Could you check a few things on this model? Use its own coordinates, in mm. A direction names the side the tool comes from. Round coordinates to 2 decimals unless told otherwise and drop trailing zeros. Write each loop counter-clockwise with the first axis right and the second up, starting at its lowest first coordinate (ties: lowest second). Pieces come first, ordered by that corner, then holes. Notation, with made-up numbers: (13.5, 22.25) -> (32.5, 22.25) arc R17 cw to (32.5, 47.25) -> close; hole circle Ø2 at (50.5, -20). An arc over 180 degrees is marked (long way). One line per question, with ' | ' between items. Start each with the question number.
1. For faces 4 (the flat face through (37, 16, 35)), 5 (the flat face through (-37.25, 18, 18)), 6 (the flat face through (-40, 18.5, 9)), which set-ups out of +Z, -Z, +X, -X, +Y, -Y let a thin tool reach every point of the face, with its end or its side?
2. Imagine slicing it at D-D, the plane y = -19. List the corners of the cut face in (x, z) for me.
3. Imagine slicing it at C-C, the plane z = 34. List the corners of the cut face in (x, y) for me.
4. If I drill on line 1 along Z through (x, y) = (-40, 17); line 2 along X through (y, z) = (17, 18); line 3 along X through (y, z) = (16, 9), over which ranges is the centre line in solid material (lowest first)? Write a range as [from, to].
5. For pin 1 Ø5 at (x, y) = (-2, 15.5) entering from +Z; pin 2 Ø8 at (x, y) = (-39.5, 17.5) entering from +Z; pin 3 Ø5 at (x, y) = (-17, 15.5) entering from -Z; pin 4 Ø1.2 at (x, z) = (28, 9) entering from -Y, each with a flat end and sliding along its axis, tell me the tip position at first contact or that it passes through.
6. Imagine slicing it at A-A, the plane x = 20.5. List the corners of the cut face in (y, z) for me, and give its area (3 significant figures).
7. Imagine slicing it at B-B, the plane z = 25.75. List the corners of the cut face in (x, y) for me.
8. Thinking about a two-plate mould opening in Y: for faces 1 (the flat face through (28, 18.5, 26)), 2 (the flat face through (44, 11, 18)), 3 (the flat face through (-7, 17, 3.25)), which applies, released by +Y, released by -Y, zero draft, split by the parting line, or undercut?
from build123d import *

# Parameters (mm, degrees)
F2_DEPTH     = 35
F4_DEPTH     = 10
F3_R         = 2
F5_DEPTH     = 0.95
F6_DEPTH     = 2.5
F7_DEPTH     = 6
F8_W         = 9
F8_H         = 9.25
F8_R         = 1.5
F8_H_2       = 6.25
F9_DEPTH     = 10
F10_DEPTH    = 10
F11_R        = 2
F12_DEPTH    = 6
F13_T1_DEPTH = 35
F13_T3_DEPTH = 35
F13_T5_DEPTH = 60
F13_T7_DEPTH = 32.9128784748


# Not quite as in the source:
# - a fillet or chamfer that OpenCascade refuses, or shapes differently, is made with other operations: its cross-section is extruded or revolved along the edge and cut away or added


with BuildPart() as f2:
    # F1 (on Top) → F2 (new body)
    with BuildSketch(Plane.XY):
        Polygon((50, -22.5), (50, 22.5), (-50, 22.5), (-50, 12.5), (40, 12.5), (40, -22.5), align=None)
    extrude(amount=F2_DEPTH)

    # F3 (on face) → F4 (cut, through all)
    with BuildSketch(Plane.XZ.offset(-12.5)):
        with BuildLine():
            Line((-37.25, 3.25), (24.75, 3.25))
            Line((24.75, 3.25), (24.75, 16.5))
            ThreePointArc((24.75, 16.5), (23.75, 17.5), (24.75, 18.5))
            Line((24.75, 18.5), (24.75, 31.75))
            Line((24.75, 31.75), (-37.25, 31.75))
            Line((-37.25, 31.75), (-37.25, 18.5))
            ThreePointArc((-37.25, 18.5), (-36.25, 17.5), (-37.25, 16.5))
            Line((-37.25, 16.5), (-37.25, 3.25))
        make_face()
        with BuildLine():
            Line((-37.25, 17.5), (-37.25, 16.5))
            ThreePointArc((-37.25, 16.5), (-36.25, 17.5), (-37.25, 18.5))
            Line((-37.25, 18.5), (-37.25, 17.5))
        make_face()
        with BuildLine():
            ThreePointArc((24.75, 18.5), (23.75, 17.5), (24.75, 16.5))
            Line((24.75, 16.5), (24.75, 17.5))
            Line((24.75, 17.5), (24.75, 18.5))
        make_face()
    extrude(amount=-F4_DEPTH, mode=Mode.SUBTRACT)

    # F3 (on face) → F5 (cut)
    with BuildSketch(Plane.XZ.offset(-12.5)):
        with BuildLine():
            Line((-43.25, 3.25), (-37.25, 3.25))
            Line((-37.25, 3.25), (-37.25, 16.5))
            Line((-37.25, 16.5), (-40.25, 16.5))
            ThreePointArc((-40.25, 16.5), (-41.25, 17.5), (-40.25, 18.5))
            Line((-40.25, 18.5), (-37.25, 18.5))
            Line((-37.25, 18.5), (-37.25, 31.75))
            Line((-37.25, 31.75), (-43.25, 31.75))
            Line((-43.25, 31.75), (-46.25, 31.75))
            Line((-46.25, 31.75), (-46.25, 3.25))
            Line((-46.25, 3.25), (-43.25, 3.25))
        make_face()
        with Locations((-40.25, 9.25)):
            Circle(F3_R, mode=Mode.SUBTRACT)
        with Locations((-40.25, 25.75)):
            Circle(F3_R, mode=Mode.SUBTRACT)
        with BuildLine():
            Line((27.75, 3.25), (30.75, 3.25))
            Line((30.75, 3.25), (33.75, 3.25))
            Line((33.75, 3.25), (33.75, 31.75))
            Line((33.75, 31.75), (30.75, 31.75))
            Line((30.75, 31.75), (24.75, 31.75))
            Line((24.75, 31.75), (24.75, 18.5))
            Line((24.75, 18.5), (27.75, 18.5))
            ThreePointArc((27.75, 18.5), (28.75, 17.5), (27.75, 16.5))
            Line((27.75, 16.5), (24.75, 16.5))
            Line((24.75, 16.5), (24.75, 3.25))
            Line((24.75, 3.25), (27.75, 3.25))
        make_face()
        with Locations((27.75, 9.25)):
            Circle(F3_R, mode=Mode.SUBTRACT)
        with Locations((27.75, 25.75)):
            Circle(F3_R, mode=Mode.SUBTRACT)
        with BuildLine():
            Line((-40.25, 16.5), (-37.25, 16.5))
            Line((-37.25, 16.5), (-37.25, 17.5))
            Line((-37.25, 17.5), (-37.25, 18.5))
            Line((-37.25, 18.5), (-40.25, 18.5))
            ThreePointArc((-40.25, 18.5), (-41.25, 17.5), (-40.25, 16.5))
        make_face()
        with BuildLine():
            Line((24.75, 17.5), (24.75, 16.5))
            Line((24.75, 16.5), (27.75, 16.5))
            ThreePointArc((27.75, 16.5), (28.75, 17.5), (27.75, 18.5))
            Line((27.75, 18.5), (24.75, 18.5))
            Line((24.75, 18.5), (24.75, 17.5))
        make_face()
    extrude(amount=-F5_DEPTH, mode=Mode.SUBTRACT)

    # F3 (on face) → F6 (cut)
    with BuildSketch(Plane.XZ.offset(-12.5)):
        with BuildLine():
            Line((-40.25, 16.5), (-37.25, 16.5))
            Line((-37.25, 16.5), (-37.25, 17.5))
            Line((-37.25, 17.5), (-37.25, 18.5))
            Line((-37.25, 18.5), (-40.25, 18.5))
            ThreePointArc((-40.25, 18.5), (-41.25, 17.5), (-40.25, 16.5))
        make_face()
        with BuildLine():
            Line((24.75, 17.5), (24.75, 16.5))
            Line((24.75, 16.5), (27.75, 16.5))
            ThreePointArc((27.75, 16.5), (28.75, 17.5), (27.75, 18.5))
            Line((27.75, 18.5), (24.75, 18.5))
            Line((24.75, 18.5), (24.75, 17.5))
        make_face()
    extrude(amount=-F6_DEPTH, mode=Mode.SUBTRACT)

    # F3 (on face) → F7 (cut)
    with BuildSketch(Plane.XZ.offset(-12.5)):
        with Locations((-40.25, 25.75)):
            Circle(F3_R)
        with Locations((-40.25, 9.25)):
            Circle(F3_R)
        with Locations((27.75, 9.25)):
            Circle(F3_R)
        with Locations((27.75, 25.75)):
            Circle(F3_R)
    extrude(amount=-F7_DEPTH, mode=Mode.SUBTRACT)

    # F8 (on face) → F9 (join, through all)
    with BuildSketch(Plane(origin=(0, 22.5, 0), x_dir=(-1, 0, 0), z_dir=(0, 1, 0))):
        with Locations((1.5, 36.375)):
            Rectangle(F8_W, F8_H)
        with Locations((1.5, 36.5)):
            Circle(F8_R, mode=Mode.SUBTRACT)
        with Locations((1.5, 0.125)):
            Rectangle(F8_W, F8_H_2)
        with Locations((1.5, 1.5)):
            Circle(F8_R, mode=Mode.SUBTRACT)
        with Locations((23.5, 36.375)):
            Rectangle(F8_W, F8_H)
        with Locations((23.5, 36.5)):
            Circle(F8_R, mode=Mode.SUBTRACT)
        with BuildLine():
            ThreePointArc((3, 36.5), (0.4393398187, 37.5606601622), (1.5000000271, 35))
            ThreePointArc((1.5000000271, 35), (2.5606601813, 35.4393398378), (3, 36.5))
        make_face()
    extrude(amount=-F9_DEPTH)

    # F8 (on face) → F10 (cut, through all)
    with BuildSketch(Plane(origin=(0, 22.5, 0), x_dir=(-1, 0, 0), z_dir=(0, 1, 0))):
        with BuildLine():
            ThreePointArc((3, 1.5), (0.4393398305, 2.560660174), (1.4999999936, 0))
            ThreePointArc((1.4999999936, 0), (2.5606601695, 0.439339826), (3, 1.5))
        make_face()
        with BuildLine():
            ThreePointArc((3, 36.5), (0.4393398187, 37.5606601622), (1.5000000271, 35))
            ThreePointArc((1.5000000271, 35), (2.5606601813, 35.4393398378), (3, 36.5))
        make_face()
    extrude(amount=-F10_DEPTH, mode=Mode.SUBTRACT)

    # F11 (on face) → F12 (cut)
    with BuildSketch(Plane.YZ.offset(50)):
        with Locations((-19, 17.5)):
            Circle(F11_R)
        with Locations((11, 17.5)):
            Circle(F11_R)
    extrude(amount=-F12_DEPTH, mode=Mode.SUBTRACT)

    # F13: fillet of radius 5 on 11 edges, made by hand

    # F13_s2 → F13_t1 (cut)
    with BuildSketch(Plane.XZ.offset(-35)):
        with BuildLine():
            ThreePointArc((-50, 30), (-48.5355339059, 33.5355339059), (-45, 35))
            Line((-45, 35), (-50, 35))
            Line((-50, 35), (-50, 30))
        make_face()
        with BuildLine():
            ThreePointArc((-45, 0), (-48.5355339059, 1.4644660941), (-50, 5))
            Line((-50, 5), (-50, 0))
            Line((-50, 0), (-45, 0))
        make_face()
        with BuildLine():
            ThreePointArc((-1, 41), (-4.5355339059, 39.5355339059), (-6, 36))
            Line((-6, 36), (-6, 41))
            Line((-6, 41), (-1, 41))
        make_face()
        with BuildLine():
            ThreePointArc((3, 36), (1.5355339059, 39.5355339059), (-2, 41))
            Line((-2, 41), (3, 41))
            Line((3, 41), (3, 36))
        make_face()
        with BuildLine():
            ThreePointArc((-28, 36), (-26.5355339059, 39.5355339059), (-23, 41))
            Line((-23, 41), (-28, 41))
            Line((-28, 41), (-28, 36))
        make_face()
        with BuildLine():
            ThreePointArc((-19, 36), (-20.4644660941, 39.5355339059), (-24, 41))
            Line((-24, 41), (-19, 41))
            Line((-19, 41), (-19, 36))
        make_face()
    extrude(amount=F13_T1_DEPTH, mode=Mode.SUBTRACT)

    # F13_s4 → F13_t3 (cut)
    with BuildSketch(Plane.YZ.offset(27.5)):
        with BuildLine():
            ThreePointArc((-22.5, 30), (-21.0355339059, 33.5355339059), (-17.5, 35))
            Line((-17.5, 35), (-22.5, 35))
            Line((-22.5, 35), (-22.5, 30))
        make_face()
        with BuildLine():
            ThreePointArc((-22.5, 5), (-21.0355339059, 1.4644660941), (-17.5, 0))
            Line((-17.5, 0), (-22.5, 0))
            Line((-22.5, 0), (-22.5, 5))
        make_face()
    extrude(amount=F13_T3_DEPTH, mode=Mode.SUBTRACT)

    # F13_s6 → F13_t5 (cut)
    with BuildSketch(Plane.XY.offset(-12.5)):
        with BuildLine():
            ThreePointArc((50, 17.5), (48.5355339059, 21.0355339059), (45, 22.5))
            Line((45, 22.5), (50, 22.5))
            Line((50, 22.5), (50, 17.5))
        make_face()
    extrude(amount=F13_T5_DEPTH, mode=Mode.SUBTRACT)

    # F13_s8 → F13_t7 (cut)
    with BuildSketch(Plane.XZ.offset(-33.9564392374)):
        with BuildLine():
            ThreePointArc((3, 0), (1.1560370926, -2.1833001327), (-1.582575695, -3))
            Line((-1.582575695, -3), (3, -3))
            Line((3, -3), (3, 0))
        make_face()
        with BuildLine():
            ThreePointArc((-1.417424305, -3), (-4.1560370926, -2.1833001327), (-6, 0))
            Line((-6, 0), (-6, -3))
            Line((-6, -3), (-1.417424305, -3))
        make_face()
    extrude(amount=F13_T7_DEPTH, mode=Mode.SUBTRACT)


solid = f2.part
Geometry results:
1) face 4: +Z, +X, +Y, -Y | face 5: +Y, -Y | face 6: -Y
2) outline: (40, 0.23) -> (50, 0.23) -> (50, 15.5) -> (44, 15.5) -> (44, 19.5) -> (50, 19.5) -> (50, 34.77) -> (40, 34.77) -> close
3) outline: (-48, 12.5) -> (40, 12.5) -> (40, -20.5) -> (50, -20.5) -> (50, 17.5) arc R5 ccw to (45, 22.5) -> (-48, 22.5) -> close
4) line 1: z = [0, 7.27], [11.23, 23.77], [27.73, 35] | line 2: x = [-50, -37.25], [24.75, 50] | line 3: x = [-50, -42.23], [-38.27, -37.25], [24.75, 25.77], [29.73, 50]
5) pin 1: stops at z = 40.97 | pin 2: stops at z = 35 | pin 3: stops at z = 0 | pin 4: stops at y = 18.5
6) outline: (12.5, 0) -> (22.5, 0) -> (22.5, 3.25) -> (12.5, 3.25) -> close; (12.5, 31.75) -> (22.5, 31.75) -> (22.5, 35) -> (12.5, 35) -> close | area: 65.0 mm2
7) outline: (-50, 12.5) -> (-46.25, 12.5) -> (-46.25, 13.45) -> (-42.25, 13.45) -> (-42.25, 18.5) -> (-38.25, 18.5) -> (-38.25, 13.45) -> (-37.25, 13.45) -> (-37.25, 22.5) -> (-50, 22.5) -> close; (24.75, 13.45) -> (25.75, 13.45) -> (25.75, 18.5) -> (29.75, 18.5) -> (29.75, 13.45) -> (33.75, 13.45) -> (33.75, 12.5) -> (40, 12.5) -> (40, -22.5) -> (50, -22.5) -> (50, 17.5) arc R5 ccw to (45, 22.5) -> (24.75, 22.5) -> close
8) face 1: released by -Y | face 2: undercut | face 3: zero draft
